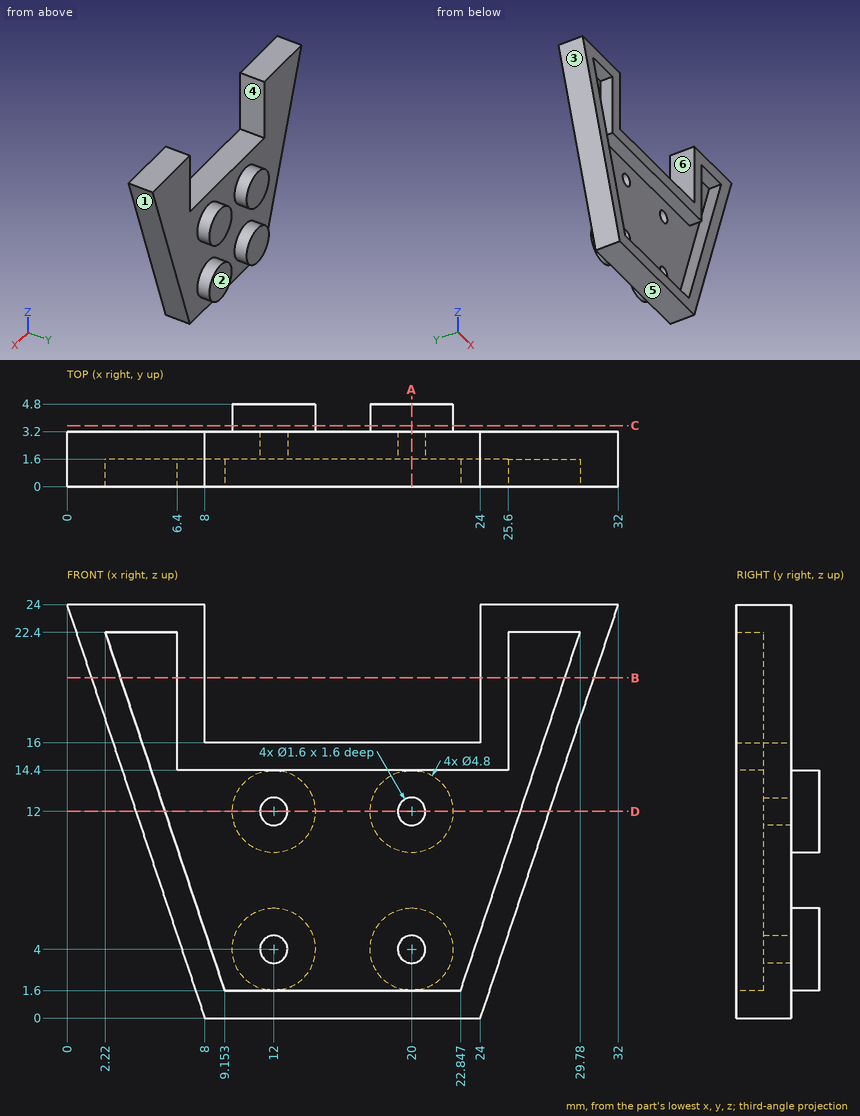
Input: dimensioned drawing with shaded views. Units: mm. Origin: part minimum x, y, z. A direction names the side the tool comes from. Give positions to 0.01 mm unless a question says otherwise; leave off trailing zeros. Loops run counter-clockwise (first coordinate to the right, second up) from the corner with the lowest first, then second, coordinate; pieces in that order, holes last. Notation, with made-up numbers: M -38,-31 L 10,-31 A16 ccw 10,-26 Z; hole C 33,20 d2. An arc over 180 degrees is marked long. Put each result on its own line as item: value. Start each with the question number.
1) Pull-direction query (X, two-part tool) for the marked faces 1, 2, 3 and 4; classes: pulls with the +X half, pulls with the -X half, needs draft (parallel to the pull), parting line crosses it, or undercut.
2) Cut plane B-B (z = 19.75). Output: boundary loops of the cut face in (x, y).
3) Ray query, line 1 along Z through (x, y) = (20, 2.65); line 2 along Z through (x, y) = (15, 1.4); line 3 along X through (y, z) = (2.9, 4). Return the intervals inside material, ascending.
4) Contact query for flat-ended pins moving along their axis: pin 1 (1.3 mm diameter, centred on x = 12, z = 4, fed in from -Y); pin 2 (1.6 mm diameter, centred on y = 1, z = 19.5, fed in from -X); pin 3 (0.8 mm diameter, centred on x = 20, z = 4.5, fed in from -Y). Output: stop coordinate, or through.
5) Cut plane D-D (z = 12). Output: boundary loops of the cut face in (x, y).
6) Access query for the marked faces 5 and 6. Directions: +Z, -Z, +X, -X, +Y, -Y. A direction counts if a zero-diameter tool reaches every point of the face in a straight line with its end or side. Return the directions, or none.
7) Cut plane A-A (x = 20). Output: boundary loops of the cut face in (y, z).
8) Cut plane C-C (y = 3.55). Output: boundary loops of the cut face in (x, z), then the cut area to 3 significant figures.
Verdict:
1. face 1: pulls with the +X half
1. face 2: needs draft
1. face 3: pulls with the -X half
1. face 4: undercut
2. outline: M 1.42,0 L 3.1,0 L 3.1,1.6 L 6.4,1.6 L 6.4,0 L 8,0 L 8,3.2 L 1.42,3.2 Z; M 24,0 L 25.6,0 L 25.6,1.6 L 28.9,1.6 L 28.9,0 L 30.58,0 L 30.58,3.2 L 24,3.2 Z
3. line 1: 0 to 3.2, 4.8 to 11.2, 12.8 to 16
3. line 2: 0 to 1.6, 14.4 to 16
3. line 3: 6.67 to 11.2, 12.8 to 19.2, 20.8 to 25.33
4. pin 1: y = 3.2
4. pin 2: x = 1.23
4. pin 3: y = 1.6
5. outline: M 4,0 L 5.69,0 L 5.69,1.6 L 11.2,1.6 L 11.2,3.2 L 12.8,3.2 L 12.8,1.6 L 19.2,1.6 L 19.2,3.2 L 20.8,3.2 L 20.8,1.6 L 26.31,1.6 L 26.31,0 L 28,0 L 28,3.2 L 22.4,3.2 L 22.4,4.8 L 17.6,4.8 L 17.6,3.2 L 14.4,3.2 L 14.4,4.8 L 9.6,4.8 L 9.6,3.2 L 4,3.2 Z
6. face 5: -Z, +X, -X, +Y, -Y
6. face 6: +Z, +Y, -Y
7. outline: M 0,0 L 3.2,0 L 3.2,1.6 L 4.8,1.6 L 4.8,6.4 L 3.2,6.4 L 3.2,9.6 L 4.8,9.6 L 4.8,14.4 L 3.2,14.4 L 3.2,16 L 0,16 L 0,14.4 L 1.6,14.4 L 1.6,12.8 L 3.2,12.8 L 3.2,11.2 L 1.6,11.2 L 1.6,4.8 L 3.2,4.8 L 3.2,3.2 L 1.6,3.2 L 1.6,1.6 L 0,1.6 Z
8. outline: C 12,4 d4.8; C 12,12 d4.8; C 20,4 d4.8; C 20,12 d4.8
8. area: 72.4 mm2
